from build123d import *

# Parameters (mm, degrees)
BOSS_EXTRUDE1_DEPTH     = 2.4
FILLET1_R               = 1
CUT_EXTRUDE1_REACH      = 32.579
CUT_EXTRUDE2_DEPTH      = 32.741278757
CUT_EXTRUDE2_DEPTH_BACK = 32.741278757
SKETCH6_R               = 1


with BuildPart() as part:
    # Sketch1 → Boss-Extrude1 (new body)
    with BuildSketch(Plane(origin=(0, 0, 0), x_dir=(1, 0, 0), z_dir=(0, 1, 0))):
        with BuildLine():
            Line((-15, 3.25), (-9.45714016, 3.25))
            ThreePointArc((-9.45714016, 3.25), (-7.071067812, 7.071067812), (-3.25, 9.45714016))
            Line((-3.25, 9.45714016), (-3.25, 15))
            ThreePointArc((-3.25, 15), (0, 18.25), (3.25, 15))
            Line((3.25, 15), (3.25, 9.45714016))
            ThreePointArc((3.25, 9.45714016), (7.071067812, 7.071067812), (9.45714016, 3.25))
            Line((9.45714016, 3.25), (15, 3.25))
            ThreePointArc((15, 3.25), (18.25, 0), (15, -3.25))
            Line((15, -3.25), (9.45714016, -3.25))
            ThreePointArc((9.45714016, -3.25), (7.071067812, -7.071067812), (3.25, -9.45714016))
            Line((3.25, -9.45714016), (3.25, -15))
            ThreePointArc((3.25, -15), (0, -18.25), (-3.25, -15))
            Line((-3.25, -15), (-3.25, -9.45714016))
            ThreePointArc((-3.25, -9.45714016), (-7.071067812, -7.071067812), (-9.45714016, -3.25))
            Line((-9.45714016, -3.25), (-15, -3.25))
            ThreePointArc((-15, -3.25), (-18.25, 0), (-15, 3.25))
        make_face()
        with BuildLine():
            Line((-15, 1.42), (-9.5, 1.42))
            ThreePointArc((-9.5, 1.42), (-8.08, 0), (-9.5, -1.42))
            Line((-9.5, -1.42), (-15, -1.42))
            ThreePointArc((-15, -1.42), (-16.42, 0), (-15, 1.42))
        make_face(mode=Mode.SUBTRACT)
        with BuildLine():
            Line((1.42, 15), (1.42, 9.5))
            ThreePointArc((1.42, 9.5), (0, 8.08), (-1.42, 9.5))
            Line((-1.42, 9.5), (-1.42, 15))
            ThreePointArc((-1.42, 15), (0, 16.42), (1.42, 15))
        make_face(mode=Mode.SUBTRACT)
        with BuildLine():
            Line((15, -1.42), (9.5, -1.42))
            ThreePointArc((9.5, -1.42), (8.08, 0), (9.5, 1.42))
            Line((9.5, 1.42), (15, 1.42))
            ThreePointArc((15, 1.42), (16.42, 0), (15, -1.42))
        make_face(mode=Mode.SUBTRACT)
        with BuildLine():
            Line((-1.42, -15), (-1.42, -9.5))
            ThreePointArc((-1.42, -9.5), (0, -8.08), (1.42, -9.5))
            Line((1.42, -9.5), (1.42, -15))
            ThreePointArc((1.42, -15), (0, -16.42), (-1.42, -15))
        make_face(mode=Mode.SUBTRACT)
    extrude(amount=BOSS_EXTRUDE1_DEPTH)

    # Fillet1
    fillet1_edges = [part.edges().sort_by_distance(p)[0] for p in [
        (-9.45714016, 1.2, -3.25),
        (-3.25, 1.2, -9.45714016),
        (3.25, 1.2, -9.45714016),
        (9.45714016, 1.2, -3.25),
        (9.45714016, 1.2, 3.25),
        (3.25, 1.2, 9.45714016),
        (-3.25, 1.2, 9.45714016),
        (-9.45714016, 1.2, 3.25),
    ]]
    fillet(fillet1_edges, radius=FILLET1_R)

    # Sketch2 → Revolve2 (revolve)
    with BuildSketch(Plane.XY, mode=Mode.PRIVATE) as revolve2_sk:
        with BuildLine():
            Line((0, 4.4), (0, 16.4))
            Line((0, 16.4), (2.9, 16.4))
            ThreePointArc((2.9, 16.4), (4.314213562, 15.814213562), (4.9, 14.4))
            Line((4.9, 14.4), (4.9, 4.4))
            Line((4.9, 4.4), (5.6, 4.4))
            Line((5.6, 4.4), (5.6, 2.4))
            Line((5.6, 2.4), (0, 2.4))
            Line((0, 2.4), (0, 4.4))
        make_face()
    revolve(revolve2_sk.sketch.rotate(Axis((0, 4.4, 0), (0, 1, 0)), 90), axis=Axis((0, 4.4, 0), (0, 1, 0)))

    # Cut-Extrude1: up to this face of the body (flat: up to its plane)
    cut_extrude1_end = Plane(part.part.faces().sort_by_distance((0, 4.4, 5.058391919))[0])
    # Sketch5 → Cut-Extrude1 (cut, up to the picked face)
    with BuildSketch(Plane(origin=(0, 16.4, 0), x_dir=(1, 0, 0), z_dir=(0, 1, 0)), mode=Mode.PRIVATE) as cut_extrude1_sk1:
        with BuildLine():
            ThreePointArc((-0.560667259, -2.845285965), (0.991858416, -2.7251086), (2.258410603, -1.819225535))
            Line((2.258410603, -1.819225535), (0.560667259, 2.845285965))
            ThreePointArc((0.560667259, 2.845285965), (-0.991858416, 2.7251086), (-2.258410603, 1.819225535))
            Line((-2.258410603, 1.819225535), (-0.560667259, -2.845285965))
        make_face()
    cut_extrude1_tool1 = split(extrude(cut_extrude1_sk1.sketch, amount=-CUT_EXTRUDE1_REACH, mode=Mode.PRIVATE), bisect_by=cut_extrude1_end, keep=Keep.BOTH, mode=Mode.PRIVATE)
    # Sketch5 → Cut-Extrude1 (cut, up to the picked face)
    with BuildSketch(Plane(origin=(0, 16.4, 0), x_dir=(1, 0, 0), z_dir=(0, 1, 0)), mode=Mode.PRIVATE) as cut_extrude1_sk2:
        with BuildLine():
            ThreePointArc((0.185903471, -4.896472189), (1.675898702, -4.604493842), (3.004981333, -3.870411759))
            Line((3.004981333, -3.870411759), (2.258410603, -1.819225535))
            ThreePointArc((2.258410603, -1.819225535), (0.991858416, -2.7251086), (-0.560667259, -2.845285965))
            Line((-0.560667259, -2.845285965), (0.185903471, -4.896472189))
        make_face()
    cut_extrude1_tool2 = split(extrude(cut_extrude1_sk2.sketch, amount=-CUT_EXTRUDE1_REACH, mode=Mode.PRIVATE), bisect_by=cut_extrude1_end, keep=Keep.BOTH, mode=Mode.PRIVATE)
    # Sketch5 → Cut-Extrude1 (cut, up to the picked face)
    with BuildSketch(Plane(origin=(0, 16.4, 0), x_dir=(1, 0, 0), z_dir=(0, 1, 0)), mode=Mode.PRIVATE) as cut_extrude1_sk3:
        with BuildLine():
            ThreePointArc((-2.258410603, 1.819225535), (-0.991858416, 2.7251086), (0.560667259, 2.845285965))
            Line((0.560667259, 2.845285965), (-0.185903471, 4.896472189))
            ThreePointArc((-0.185903471, 4.896472189), (-1.675898702, 4.604493842), (-3.004981333, 3.870411759))
            Line((-3.004981333, 3.870411759), (-2.258410603, 1.819225535))
        make_face()
    cut_extrude1_tool3 = split(extrude(cut_extrude1_sk3.sketch, amount=-CUT_EXTRUDE1_REACH, mode=Mode.PRIVATE), bisect_by=cut_extrude1_end, keep=Keep.BOTH, mode=Mode.PRIVATE)
    add(cut_extrude1_tool1.solids().sort_by(Axis((0, 16.4, 0), (0, -1, 0)))[0], mode=Mode.SUBTRACT)
    add(cut_extrude1_tool2.solids().sort_by(Axis((1.296647, 16.4, 3.562508), (0, -1, 0)))[0], mode=Mode.SUBTRACT)
    add(cut_extrude1_tool3.solids().sort_by(Axis((-1.296647, 16.4, -3.562508), (0, -1, 0)))[0], mode=Mode.SUBTRACT)

    # Sketch6 → Cut-Extrude2 (cut, two sides: drawn at the far end of the back side and taken through both)
    with BuildSketch(Plane(origin=(1.409538931, 0, -0.513030215), x_dir=(0.3420201433256665, 0, 0.9396926207859093), z_dir=(-0.9396926207859092, 0, 0.34202014332566644)).offset(-CUT_EXTRUDE2_DEPTH_BACK)):
        with Locations((0, 10)):
            Circle(SKETCH6_R)
    extrude(amount=CUT_EXTRUDE2_DEPTH + CUT_EXTRUDE2_DEPTH_BACK, mode=Mode.SUBTRACT)


solid = part.part
The listing builds one solid part. Answer for the finished solid, in the listing's coordinates (mm). A direction names the side the tool comes from. Coordinates: 2 decimals unless noted, no trailing zeros. Write each loop counter-clockwise with the first axis right and the second up, starting at its lowest first coordinate (ties: lowest second). Pieces come first, ordered by that corner, then holes. Notation, with made-up numbers: M 5.5,71.5 L 64.5,71.5 A8 cw 64.5,81.5 Z; hole C 58,42 d4. An arc over 180 degrees is marked long. Use one line per item in the form item = value.
Item 1: Find the intervals of material crossed by probe 1 along Y at (x, z) = (16, -2.5); probe 2 along Y at (x, z) = (1, 1); probe 3 along Z at (x, y) = (4, 9.25), in increasing order.
Model answer:
probe_1 = 0 to 2.4
probe_2 = 0 to 4.4
probe_3 = -2.83 to -2.16, -0.75 to 2.83
Item 2: For faces 4 (the face through (1.42, 1, -12)), 5 (the face through (-0.246, 3.386, 5.595)), 6 (the face through (3.25, 1, 13)), 7 (the face through (3.25, 1, -13)), determine the directions among +Z, -Z, +X, -X, +Y, -Y from which every point of the face is accessible in a straight line to the end or side of a thin tool.
Model answer:
face_4 = +Y, -Y
face_5 = +Y
face_6 = +Z, +X, +Y, -Y
face_7 = -Z, +X, +Y, -Y
Item 3: The mould has two halves that part along Z. Classify faces 1 (the face through (8.08, 1.18, 0.03)), 2 (the face through (-0.07, 1.18, -18.25)), 3 (the face through (-7.03, 1.18, 7.11)): released by +Z, released by -Z, zero draft, split by the parting line, or undercut.
Model answer:
face_1 = undercut
face_2 = released by -Z
face_3 = released by +Z
Item 4: Find section C-C, the plane z = -7.5. Give the vertices of the cut face in (x, y), plus the area to 3 significant figures.
Model answer:
outline = M -6.61,0 L 6.61,0 L 6.61,2.4 L -6.61,2.4 Z
area = 31.7 mm2
Item 5: Find section D-D, the plane x = 7.5. Give the vertices of the cut face in (y, z).
Model answer:
outline = M 0,-6.61 L 2.4,-6.61 L 2.4,6.61 L 0,6.61 Z
Item 6: Given P1, Ø0.7, axis at y = 1, z = -13.5, coming from the +X side; P2, Ø2.5, axis at x = -13.5, y = 1.5, coming from the -Z side; P3, Ø2.5, axis at y = 1, z = -12, coming from the -X side, each flat-ended and moving along its own axis, determine where each tip first touches the part or whether it passes through.
Model answer:
P1 = 3.25
P2 = -3.25
P3 = -3.25
Item 7: Find section A-A, the plane z = 14. Give the vertices of the cut face in (x, y).
Model answer:
outline = M -3.25,0 L -1.42,0 L -1.42,2.4 L -3.25,2.4 Z; M 1.42,0 L 3.25,0 L 3.25,2.4 L 1.42,2.4 Z
Item 8: Find section B-B, the plane x = 13. Give the vertices of the cut face in (y, z), plus the area to 3 significant figures.
Model answer:
outline = M 0,-3.25 L 2.4,-3.25 L 2.4,-1.42 L 0,-1.42 Z; M 0,1.42 L 2.4,1.42 L 2.4,3.25 L 0,3.25 Z
area = 8.78 mm2
